Can you work these out from the model? Positions are in its coordinate system, mm. Face numbers are marked on the shaded views. A direction names the side the tool comes from. Round coordinates to 2 decimals unless told otherwise and drop trailing zeros. Loops run counter-clockwise (first coordinate to the right, second up) from the corner with the lowest first, then second, coordinate; pieces in that order, holes last.
(1) Will these pins go through, and if not, where does the flat tip stop? pin 1 Ø2 at (y, z) = (-0.5, 4.5) entering from +X; pin 2 Ø1.5 at (y, z) = (9.5, 1) entering from +X.
(2) I want a section at D-D on z = 5.5. Write out the boundary of the cut face in (x, y).
(3) I want a section at A-A on y = 0. Write out the boundary of the cut face in (x, z), plus the area to 3 significant figures.
(4) If I drill on line 1 along Z through (x, y) = (1.5, 7.75); line 2 along Y through (x, z) = (-0.25, 1.75); line 3 along Z through (x, y) = (9.25, -5), over which ranges is the centre line in solid material (lowest first)?
(5) I want a section at C-C on z = 1.75. Write out the boundary of the cut face in (x, y), plus the area to 3 significant figures.
(6) Which directions (+Z, -Z, +X, -X, +Y, -Y) give clear straight access to the entire face, cutting with the end or side of a thin tool? Please do the marked faces 1 and 2.
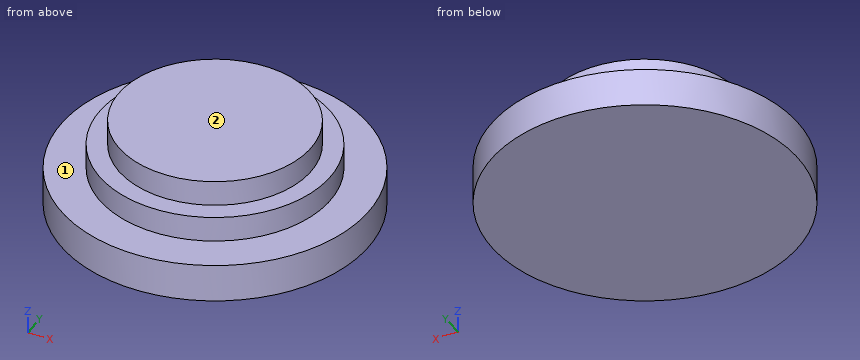
from build123d import *

# Parameters (mm, degrees)
SKETCH001_R      = 9
EXTRUDE001_DEPTH = 5
SKETCH004_R      = 12
EXTRUDE004_DEPTH = 3
SKETCH_R         = 7.5
EXTRUDE_DEPTH    = 7


with BuildPart() as extrude001:
    # Sketch001 → Extrude001 (new body)
    with BuildSketch(Plane.XY):
        Circle(SKETCH001_R)
    extrude(amount=EXTRUDE001_DEPTH)


with BuildPart() as extrude004:
    # Sketch004 → Extrude004 (new body)
    with BuildSketch(Plane.XY):
        Circle(SKETCH004_R)
    extrude(amount=EXTRUDE004_DEPTH)


with BuildPart() as fusion:
    # Sketch → Extrude (new body)
    with BuildSketch(Plane.XY):
        Circle(SKETCH_R)
    extrude(amount=EXTRUDE_DEPTH)

    # Fusion: union Extrude001, Extrude004
    add(extrude001.part)
    add(extrude004.part)


solid = fusion.part
Filled sheet:
1. pin 1: stops at x = 9
1. pin 2: stops at x = 8.21
2. outline: circle Ø15 at (0, 0)
3. outline: (-12, 0) - (12, 0) - (12, 3) - (9, 3) - (9, 5) - (7.5, 5) - (7.5, 7) - (-7.5, 7) - (-7.5, 5) - (-9, 5) - (-9, 3) - (-12, 3) - close
3. area: 138 mm2
4. line 1: z = 0 to 5
4. line 2: y = -12 to 12
4. line 3: z = 0 to 3
5. outline: circle Ø24 at (0, 0)
5. area: 452 mm2
6. face 1: +Z
6. face 2: +Z, +X, -X, +Y, -Y
